Read the model definition and answer for the solid it produces. Units are mm, in the model's axes. A direction names the side the tool comes from. Coordinates: 2 decimals unless noted, no trailing zeros. Write each loop counter-clockwise with the first axis right and the second up, starting at its lowest first coordinate (ties: lowest second). Pieces come first, ordered by that corner, then holes.
(1) Given pin 1 (2 mm diameter, centred on x = -3, y = 2, fed in from -Z); pin 2 (8.5 mm diameter, centred on y = 0, z = -4.825, fed in from -X); pin 3 (3 mm diameter, centred on x = -0.5, y = 8, fed in from -Z); pin 4 (0.5 mm diameter, centred on y = 0.5, z = 5.5, fed in from -X), each flat-ended and moving along its own axis, determine where each tip first touches the part or whether it passes through.
(2) Section B-B on z = 6.5 is taken. Write down the section's boundary in (x, y).
(3) Section A-A on x = -2 is taken. State how many separate pieces and enclosed holes the cut face has, then the cut area to 3 significant figures.
(4) Section C-C on y = 8.5 is taken. Write down the section's boundary in (x, z), then the cut area to 3 significant figures.
(5) Which of the six approach directions +Z, -Z, +X, -X, +Y, -Y give full straight-line access (tool end or side, diameter ignored) to faces 4 (the flat face through (0, -7, 10)), 5 (the flat face through (-2.5, 1.1, 5.5)), 6 (the cylindrical face through (0.035, 2.065, 6.699))?
(6) The mould has two halves that part along Y. Classify faces 1 (the flat face through (0, 8, 0)), 2 (the flat face through (0, -7.5, 8)), 3 (the flat face through (0, -10, 6)): +Y half, -Y half, draft (parallel to the pull), parting line (faces both ways), or undercut.
(7) Find the intervals of material crossed by probe 1 along Y at (x, z) = (-3.25, 8.5); probe 2 along Z at (x, y) = (-3.75, 1); probe 3 along Z at (x, y) = (1.75, 1.5), in increasing order.
from build123d import *

# Parameters (mm, degrees)
F0_W         = 10
F0_H         = 20
F1_DEPTH     = 5
F2_W         = 10
F2_H         = 2.5
F3_DEPTH     = 7
F4_W         = 10
F4_H         = 2
F5_DEPTH     = 1
F6_W         = 5
F6_H         = 2.5
F7_DEPTH     = 2
F8_R         = 1
F9_W         = 6.5
F9_H         = 1.5
F10_DEPTH    = 10.001
F12_DEPTH    = 5
F13_R        = 4.825
F14_DEPTH    = 10.001
F15_T1_DEPTH = 10


# Not quite as in the source:
# - a fillet or chamfer that OpenCascade refuses, or shapes differently, is made with other operations: its cross-section is extruded or revolved along the edge and cut away or added


with BuildPart() as f1:
    # F0 (on Top) → F1 (new body)
    with BuildSketch(Plane.XY):
        Rectangle(F0_W, F0_H)
    extrude(amount=F1_DEPTH)

    # F2 (on face) → F3 (join)
    with BuildSketch(Plane.XY.offset(5)):
        with Locations((0, -8.75)):
            Rectangle(F2_W, F2_H)
        with Locations((0, 8.75)):
            Rectangle(F2_W, F2_H)
    extrude(amount=F3_DEPTH)

    # F4 (on face) → F5 (join)
    with BuildSketch(Plane(origin=(0, -7.5, 0), x_dir=(-1, 0, 0), z_dir=(0, 1, 0))):
        with Locations((0, 11)):
            Rectangle(F4_W, F4_H)
    extrude(amount=F5_DEPTH)

    # F6 (on face) → F7 (join)
    with BuildSketch(Plane.XY.offset(5)):
        with Locations((0, 1.1)):
            Rectangle(F6_W, F6_H)
    extrude(amount=F7_DEPTH)

    # F8
    f8_edges = [f1.edges().sort_by_distance(p)[0] for p in [
        (0, 7.5, 5),
        (0, -7.5, 5),
        (0, 10, 0),
        (0, -10, 0),
        (5, -10, 6),
        (-5, -10, 6),
        (5, 10, 6),
        (-5, 10, 6),
        (2.5, 1.1, 7),
        (0, 2.35, 7),
        (-2.5, 1.1, 7),
        (0, -0.15, 7),
    ]]
    fillet(f8_edges, radius=F8_R)

    # F9 (on face) → F10 (cut, through all)
    with BuildSketch(Plane.YZ.offset(5)):
        with Locations((0, 1.25)):
            Rectangle(F9_W, F9_H)
    extrude(amount=-F10_DEPTH, mode=Mode.SUBTRACT)

    # F11 (on Right) → F12 (join, symmetric)
    with BuildSketch(Plane.YZ):
        with BuildLine():
            Line((4.0896210093, 0), (0, 0))
            Line((0, 0), (-4.0896210093, 0))
            ThreePointArc((-4.0896210093, 0), (0, -11.15), (4.0896210093, 0))
        make_face()
        with BuildLine():
            ThreePointArc((0, 0), (3.4117902192, -1.4132097808), (4.825, -4.825))
            ThreePointArc((4.825, -4.825), (-3.4117902192, -8.2367902192), (0, 0))
        make_face(mode=Mode.SUBTRACT)
        with BuildLine():
            ThreePointArc((0, 0), (-3.4117902192, -8.2367902192), (4.825, -4.825))
            ThreePointArc((4.825, -4.825), (3.4117902192, -1.4132097808), (0, 0))
        make_face()
    extrude(amount=F12_DEPTH, both=True)

    # F13 (on face) → F14 (cut, through all)
    with BuildSketch(Plane(origin=(-5, 0, 0), x_dir=(0, -1, 0), z_dir=(-1, 0, 0))):
        with Locations((0, -4.825)):
            Circle(F13_R)
    extrude(amount=-F14_DEPTH, mode=Mode.SUBTRACT)

    # F15: fillet of radius 1 on 4 edges, made by hand

    # F15_s2 → F15_t1 (join)
    with BuildSketch(Plane.YZ.offset(-5)):
        with BuildLine():
            ThreePointArc((-6.2469992797, 0), (-5.3745933247, -0.5112179935), (-5.3941666135, -1.5221843003))
            ThreePointArc((-5.3941666135, -1.5221843003), (-4.8025845312, -0.7090788613), (-4.0896210093, 0))
            Line((-4.0896210093, 0), (-6.2469992797, 0))
        make_face()
        with BuildLine():
            ThreePointArc((6.2469992797, 0), (5.3745933247, -0.5112179935), (5.3941666135, -1.5221843003))
            ThreePointArc((5.3941666135, -1.5221843003), (4.8025845312, -0.7090788613), (4.0896210093, 0))
            Line((4.0896210093, 0), (6.2469992797, 0))
        make_face()
    extrude(amount=F15_T1_DEPTH)

    # F15_s3 → F15_t4 (revolve, cut)
    with BuildSketch(Plane.XY.offset(-4.825)):
        with BuildLine():
            ThreePointArc((-5, -5.825), (-4.7071067812, -5.1178932188), (-4, -4.825))
            Line((-4, -4.825), (-5, -4.825))
            Line((-5, -4.825), (-5, -5.825))
        make_face()
    revolve(axis=Axis((-5, 0, -4.825), (-1, 0, 0)), mode=Mode.SUBTRACT)

    # F15_s5 → F15_t6 (revolve, cut)
    with BuildSketch(Plane.XY.offset(-4.825)):
        with BuildLine():
            ThreePointArc((5, -5.825), (4.7071067812, -5.1178932188), (4, -4.825))
            Line((4, -4.825), (5, -4.825))
            Line((5, -4.825), (5, -5.825))
        make_face()
    revolve(axis=Axis((5, 0, -4.825), (-1, 0, 0)), mode=Mode.SUBTRACT)


solid = f1.part
Response:
1. pin 1: stops at z = -11.07
1. pin 2: passes through
1. pin 3: stops at z = 0
1. pin 4: stops at x = -2.5
2. outline: (-5, -9) arc R1 ccw to (-4, -10) - (4, -10) arc R1 ccw to (5, -9) - (5, -7.5) - (-5, -7.5) - close; (-5, 7.5) - (5, 7.5) - (5, 9) arc R1 ccw to (4, 10) - (-4, 10) arc R1 ccw to (-5, 9) - close; (-2.37, -0.02) - (2.37, -0.02) - (2.37, 2.22) - (-2.37, 2.22) - close
3. separate pieces: 1
3. enclosed holes: 2
3. area: 178 mm2
4. outline: (-5, 0) - (5, 0) - (5, 12) - (-5, 12) - close
4. area: 120 mm2
5. face 4: +X, -X
5. face 5: +Z, -X
5. face 6: +Z, +X, -X
6. face 1: draft
6. face 2: undercut
6. face 3: -Y half
7. probe 1: y = -10 to -7.5, 7.5 to 10
7. probe 2: z = -11.07 to -9.55, -0.1 to 0.5, 2 to 5
7. probe 3: z = -10.97 to -9.41, -0.24 to 0.5, 2 to 6.97
